from build123d import *

# Parameters (mm, degrees)
SKETCH_R      = 30.15
SKETCH_R_2    = 24.15
PAD_DEPTH     = 48
SKETCH001_R   = 24
SKETCH001_R_2 = 9.5
PAD001_DEPTH  = 10


with BuildPart() as part:
    # Sketch → Pad (new body)
    with BuildSketch(Plane.XY):
        Circle(SKETCH_R)
        Circle(SKETCH_R_2, mode=Mode.SUBTRACT)
    extrude(amount=PAD_DEPTH)

    # Sketch001 → Pad001 (join)
    with BuildSketch(Plane.XZ.offset(-5)):
        with Locations((50, 24.15)):
            Circle(SKETCH001_R)
        with Locations((50, 24.15)):
            Circle(SKETCH001_R_2, mode=Mode.SUBTRACT)
    extrude(amount=PAD001_DEPTH)


solid = part.part
Verification items for the finished model (mm, model axes). A direction names the side the tool comes from. Give positions to 0.01 mm unless a question says otherwise; leave off trailing zeros. Write each loop counter-clockwise with the first axis right and the second up, starting at its lowest first coordinate (ties: lowest second). Pieces come first, ordered by that corner, then holes.
(1) Cross-section at B-B (x = 50). Enter the section's corners in (y, z), plus the area to 3 significant figures.
(2) Cross-section at A-A (z = 24.15). Enter the section's corners in (x, y).
(3) Access from +Z, -Z, +X, -X, +Y, -Y to the whole of each face (thin tool, end or side, straight path). Record for faces 3 (the face through (52, 5, 14)), 4 (the face through (0, 25, 0)), 5 (the face through (52, -5, 14)).
(4) Cross-section at C-C (y = 2.5). Enter the section's corners in (x, z).
(5) Material ranges on line 1 (Z direction, x = 50, y = 2.5); line 2 (Y direction, x = 0, z = 32.5); line 3 (X direction, y = 17, z = 26), recorded low to high.
(6) Gauge pin test, flat ends, axial feed: pin 1 (8 mm diameter, centred on x = 39, y = 8.5, fed in from -Z); pin 2 (2 mm diameter, centred on x = 11, z = 18.5, fed in from -Y); pin 3 (2 mm diameter, centred on x = 32, z = 7, fed in from -Y). Record the tip position at first contact, or that the pin passes through.
(7) Mould release check, pull along X, two halves, no side actions. Record for faces 1 (the face through (-24.127, 1.062, 23.664)), 2 (the face through (0, 25, 48)): +X half, -X half, draft (parallel to the pull), parting line (faces both ways), or undercut.
(8) Cross-section at D-D (y = -22). Enter the section's corners in (x, z).
Worked out:
1. outline: (-5, 0.15) - (5, 0.15) - (5, 14.65) - (-5, 14.65) - close; (-5, 33.65) - (5, 33.65) - (5, 48.15) - (-5, 48.15) - close
1. area: 290 mm2
2. outline: (29.73, -5) - (40.5, -5) - (40.5, 5) - (29.73, 5) arc R30.15 ccw (long way) to start; (59.5, -5) - (74, -5) - (74, 5) - (59.5, 5) - close; hole circle Ø48.3 at (0, 0)
3. face 3: +Z, -Z, +X, +Y
3. face 4: -Z, +X, -X, +Y, -Y
3. face 5: +Z, -Z, +X, -Y
4. outline: (-30.05, 0) - (-24.02, 0) - (-24.02, 48) - (-30.05, 48) - close; (24.02, 0) - (30.05, 0) - (30.05, 10.81) arc R24 ccw (long way) to (30.05, 37.49) - (30.05, 48) - (24.02, 48) - close; hole circle Ø19 at (50, 24.15)
5. line 1: z = 0.15 to 14.65, 33.65 to 48.15
5. line 2: y = -30.15 to -24.15, 24.15 to 30.15
5. line 3: x = -24.9 to -17.15, 17.15 to 24.9
6. pin 1: stops at z = 1.93
6. pin 2: stops at y = -28.44
6. pin 3: stops at y = -5
7. face 1: undercut
7. face 2: draft
8. outline: (-20.62, 0) - (-9.96, 0) - (-9.96, 48) - (-20.62, 48) - close; (9.96, 0) - (20.62, 0) - (20.62, 48) - (9.96, 48) - close
